Drawing for the job (mm, zero at the part's lowest x, y, z). A direction names the side the tool comes from. Coordinates: 2 decimals unless noted, no trailing zeros. Order: outer loops, then holes, each group sorted by start corner. A loop starts at its lowest first (then second) coordinate and runs counter-clockwise, first axis right, second up. Notation, with made-up numbers: (49.5, -26.5) - (61.5, -26.5) arc R12 ccw to (61.5, -3.5) - close; hole circle Ø8 at (1.25, 40.25). An arc over 180 degrees is marked (long way). Put each result on its own line as item: value. Start each with the question number.
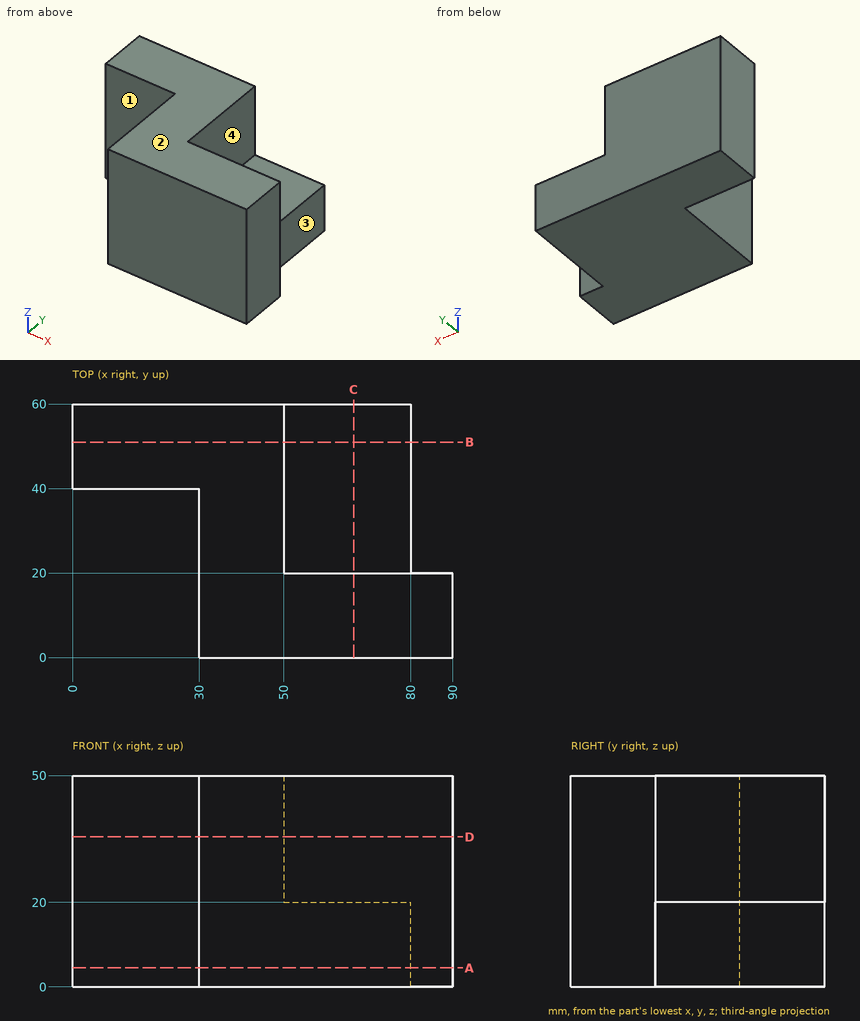
Item 1: 3-axis set-ups, long thin cutter, end or side, ignore diameter. For the marked faces 1, 2, 3 and 4: which of +Z, -Z, +X, -X, +Y, -Y reach the whole face in a straight line?
Item 2: Flat gauge pins, fed straight in: pin 1 Ø15 at (x, z) = (19, 21) entering from -Y; pin 2 Ø6 at (y, z) = (52, 27.5) entering from +X; pin 3 Ø12 at (x, z) = (75.5, 32) entering from +Y; pin 4 Ø10 at (x, y) = (14, 33.5) entering from +Z. Where does each tip first touch, or does it go through?
Item 3: Slice it at A-A, the plane z = 4.5. Give the cut face in (x, y), plus the area to 3 significant figures.
Item 4: Slice it at D-D, the plane z = 35.5. Give the cut face in (x, y).
Item 5: Wall check: line 1 along Y through (x, z) = (7, 34); line 2 along X through (y, z) = (21, 47); line 3 along X through (y, z) = (11, 4.5). Give the ranges that are in metal, low to high.
Item 6: Slice it at B-B, the plane y = 51. Give the cut face in (x, z), plus the area to 3 significant figures.
Item 7: Slice it at C-C, the plane x = 66.5. Give the cut face in (y, z).
Here are the results:
1. face 1: +Z, -Z, -X, -Y
1. face 2: +Z, +X, -X, +Y, -Y
1. face 3: +Z, -Z, +X, +Y
1. face 4: +Z, +X, +Y
2. pin 1: stops at y = 40
2. pin 2: stops at x = 50
2. pin 3: stops at y = 20
2. pin 4: passes through
3. outline: (0, 40) - (30, 40) - (30, 0) - (90, 0) - (90, 20) - (80, 20) - (80, 60) - (0, 60) - close
3. area: 3,800 mm^2
4. outline: (0, 40) - (30, 40) - (30, 0) - (90, 0) - (90, 20) - (50, 20) - (50, 60) - (0, 60) - close
5. line 1: y = 40 to 60
5. line 2: x = 30 to 50
5. line 3: x = 30 to 90
6. outline: (0, 0) - (80, 0) - (80, 20) - (50, 20) - (50, 50) - (0, 50) - close
6. area: 3,100 mm^2
7. outline: (0, 0) - (60, 0) - (60, 20) - (20, 20) - (20, 50) - (0, 50) - close
